Could you check a few things on this model? Use its own coordinates, in mm. A direction names the side the tool comes from. Coordinates: 2 decimals unless noted, no trailing zeros. Write each loop counter-clockwise with the first axis right and the second up, starting at its lowest first coordinate (ties: lowest second). Pieces come first, ordered by that corner, then holes. Notation, with made-up numbers: (-35.75, 61.25) - (-30.75, 61.25) arc R5 ccw to (-30.75, 68.25) - close; hole circle Ø6 at (-18, -33). An arc over 180 degrees is marked (long way). Answer as a JSON object with one key per item and string values. Group by question number.
1) Will these pins go through, and if not, where does the flat tip stop? pin 1 Ø12 at (x, y) = (11.5, 9.5) entering from -Z; pin 2 Ø3.5 at (x, y) = (-19, -12) entering from +Z.
2) If we section it at B-B (y = 12.5): Write out the boundary of the cut face in (x, z), plus the area to 3 significant figures.
3) On a 3-axis mill with a long thin cutter (end or side, diameter ignored), from which of +Z, -Z, +X, -X, +Y, -Y can I reach the whole of each face in a straight line? I mean faces 1 (the cylindrical face through (-17.5, 4.07, 4.93)), 2 (the cylindrical face through (16.5, 4.1, 12.5)). Say none if no direction works.
4) Please list where these lines run through material, in increasing order: line 1 along Y through (x, z) = (-12.5, 6.5); line 2 along Y through (x, z) = (-19, 5.5); line 3 along X through (y, z) = (5, 6).
5) If we section it at C-C (z = 4.5): State how many separate pieces and enclosed holes the cut face has, plus the area to 3 significant figures.
6) If we section it at A-A (x = -19): Write out the boundary of the cut face in (y, z), plus the area to 3 significant figures.
7) We'd pull the mould along Y, two halves only. Please class faces 3 (the flat face through (-19, 2, 10)), 4 (the flat face through (0, 0, 0)), 5 (the flat face through (0, -25, 7)): released by +Y, released by -Y, zero draft, split by the parting line, or undercut.
```python
from build123d import *

# Parameters (mm, degrees)
SKETCH1_W           = 50
SKETCH1_H           = 50
BOSS_EXTRUDE1_DEPTH = 15
CUT_EXTRUDE1_REACH  = 40.406
SKETCH2_R           = 1.5
SKETCH3_R           = 2.5
CUT_EXTRUDE2_DEPTH  = 5
CUT_EXTRUDE3_REACH  = 40.406
SKETCH4_R           = 1.5


with BuildPart() as part:
    # Sketch1 → Boss-Extrude1 (new body)
    with BuildSketch(Plane.XY):
        Rectangle(SKETCH1_W, SKETCH1_H)
    extrude(amount=BOSS_EXTRUDE1_DEPTH)

    # Sketch2 → Cut-Extrude1 (cut, up to next)
    with BuildSketch(Plane(origin=(0, 0, 0), x_dir=(-1, 0, 0), z_dir=(0, 0, -1)), mode=Mode.PRIVATE) as cut_extrude1_sk1:
        with Locations((-19, 4)):
            Circle(SKETCH2_R)
    cut_extrude1_tool1 = extrude(cut_extrude1_sk1.sketch, amount=-CUT_EXTRUDE1_REACH, mode=Mode.PRIVATE) & part.part
    # Sketch2 → Cut-Extrude1 (cut, up to next)
    with BuildSketch(Plane(origin=(0, 0, 0), x_dir=(-1, 0, 0), z_dir=(0, 0, -1)), mode=Mode.PRIVATE) as cut_extrude1_sk2:
        with Locations((-19, -12)):
            Circle(SKETCH2_R)
    cut_extrude1_tool2 = extrude(cut_extrude1_sk2.sketch, amount=-CUT_EXTRUDE1_REACH, mode=Mode.PRIVATE) & part.part
    # Sketch2 → Cut-Extrude1 (cut, up to next)
    with BuildSketch(Plane(origin=(0, 0, 0), x_dir=(-1, 0, 0), z_dir=(0, 0, -1)), mode=Mode.PRIVATE) as cut_extrude1_sk3:
        with Locations((19, -12)):
            Circle(SKETCH2_R)
    cut_extrude1_tool3 = extrude(cut_extrude1_sk3.sketch, amount=-CUT_EXTRUDE1_REACH, mode=Mode.PRIVATE) & part.part
    # Sketch2 → Cut-Extrude1 (cut, up to next)
    with BuildSketch(Plane(origin=(0, 0, 0), x_dir=(-1, 0, 0), z_dir=(0, 0, -1)), mode=Mode.PRIVATE) as cut_extrude1_sk4:
        with Locations((19, 4)):
            Circle(SKETCH2_R)
    cut_extrude1_tool4 = extrude(cut_extrude1_sk4.sketch, amount=-CUT_EXTRUDE1_REACH, mode=Mode.PRIVATE) & part.part
    add(cut_extrude1_tool1.solids().sort_by_distance((19, 4, 0))[0], mode=Mode.SUBTRACT)
    add(cut_extrude1_tool2.solids().sort_by_distance((19, -12, 0))[0], mode=Mode.SUBTRACT)
    add(cut_extrude1_tool3.solids().sort_by_distance((-19, -12, 0))[0], mode=Mode.SUBTRACT)
    add(cut_extrude1_tool4.solids().sort_by_distance((-19, 4, 0))[0], mode=Mode.SUBTRACT)

    # Sketch3 → Cut-Extrude2 (cut)
    with BuildSketch(Plane.XY.offset(15)):
        with Locations((-19, 4)):
            Circle(SKETCH3_R)
        with Locations((-19, -12)):
            Circle(SKETCH3_R)
        with Locations((19, 4)):
            Circle(SKETCH3_R)
        with Locations((19, -12)):
            Circle(SKETCH3_R)
    extrude(amount=-CUT_EXTRUDE2_DEPTH, mode=Mode.SUBTRACT)

    # Sketch4 → Cut-Extrude3 (cut, up to next)
    with BuildSketch(Plane.XY.offset(15), mode=Mode.PRIVATE) as cut_extrude3_sk1:
        with Locations((-12.5, -12.5)):
            Circle(SKETCH4_R)
    cut_extrude3_tool1 = extrude(cut_extrude3_sk1.sketch, amount=-CUT_EXTRUDE3_REACH, mode=Mode.PRIVATE) & part.part
    # Sketch4 → Cut-Extrude3 (cut, up to next)
    with BuildSketch(Plane.XY.offset(15), mode=Mode.PRIVATE) as cut_extrude3_sk2:
        with Locations((-12.5, 12.5)):
            Circle(SKETCH4_R)
    cut_extrude3_tool2 = extrude(cut_extrude3_sk2.sketch, amount=-CUT_EXTRUDE3_REACH, mode=Mode.PRIVATE) & part.part
    # Sketch4 → Cut-Extrude3 (cut, up to next)
    with BuildSketch(Plane.XY.offset(15), mode=Mode.PRIVATE) as cut_extrude3_sk3:
        with Locations((12.5, -12.5)):
            Circle(SKETCH4_R)
    cut_extrude3_tool3 = extrude(cut_extrude3_sk3.sketch, amount=-CUT_EXTRUDE3_REACH, mode=Mode.PRIVATE) & part.part
    # Sketch4 → Cut-Extrude3 (cut, up to next)
    with BuildSketch(Plane.XY.offset(15), mode=Mode.PRIVATE) as cut_extrude3_sk4:
        with Locations((12.5, 12.5)):
            Circle(SKETCH4_R)
    cut_extrude3_tool4 = extrude(cut_extrude3_sk4.sketch, amount=-CUT_EXTRUDE3_REACH, mode=Mode.PRIVATE) & part.part
    add(cut_extrude3_tool1.solids().sort_by_distance((-12.5, -12.5, 15))[0], mode=Mode.SUBTRACT)
    add(cut_extrude3_tool2.solids().sort_by_distance((-12.5, 12.5, 15))[0], mode=Mode.SUBTRACT)
    add(cut_extrude3_tool3.solids().sort_by_distance((12.5, -12.5, 15))[0], mode=Mode.SUBTRACT)
    add(cut_extrude3_tool4.solids().sort_by_distance((12.5, 12.5, 15))[0], mode=Mode.SUBTRACT)


solid = part.part
```
Here are the results:
{
 "1": {"pin 1": "stops at z = 0", "pin 2": "stops at z = 10"},
 "2": {"outline": "(-25, 0) - (-14, 0) - (-14, 15) - (-25, 15) - close; (-11, 0) - (11, 0) - (11, 15) - (-11, 15) - close; (14, 0) - (25, 0) - (25, 15) - (14, 15) - close", "area": "660 mm²"},
 "3": {"face 1": "+Z, -Z", "face 2": "+Z"},
 "4": {"line 1": "y = -25 to -14, -11 to 11, 14 to 25", "line 2": "y = -25 to -13.5, -10.5 to 2.5, 5.5 to 25", "line 3": "x = -25 to -20.12, -17.88 to 17.88, 20.12 to 25"},
 "5": {"separate pieces": "1", "enclosed holes": "8", "area": "2,440 mm²"},
 "6": {"outline": "(-25, 0) - (-13.5, 0) - (-13.5, 10) - (-14.5, 10) - (-14.5, 15) - (-25, 15) - close; (-10.5, 0) - (2.5, 0) - (2.5, 10) - (1.5, 10) - (1.5, 15) - (-9.5, 15) - (-9.5, 10) - (-10.5, 10) - close; (5.5, 0) - (25, 0) - (25, 15) - (6.5, 15) - (6.5, 10) - (5.5, 10) - close", "area": "640 mm²"},
 "7": {"face 3": "undercut", "face 4": "zero draft", "face 5": "released by -Y"}
}
